Verification items for the finished model (mm, model axes). A direction names the side the tool comes from. Give positions to 0.01 mm unless a question says otherwise; leave off trailing zeros. Order: outer loops, then holes, each group sorted by start corner. A loop starts at its lowest first (then second) coordinate and runs counter-clockwise, first axis right, second up.
(1) Sectioned sample at D-D on z = -23. Record the cut outline in (x, y).
(2) Sectioned sample at B-B on y = 0. Record the cut outline in (x, z), plus the area to 3 significant figures.
(3) Sectioned sample at C-C on z = -9. Record the cut outline in (x, y).
(4) Scan lines: L1, parallel to Y at x = -11.6, z = -8; L2, parallel to Y at x = -10.05, z = -8.5; L3, parallel to Y at x = -11.4, z = 1. Record each from-to range of solid material in increasing order.
(5) Mould release check, pull along Z, two halves, no side actions. Record for faces 1 (the face through (-11, -11, -6.201)), 2 (the face through (-11, 0, -37)), 3 (the face through (-11, 9.615, 25)), 4 (the face through (-10, 0, 38)): pulls with the +Z half, pulls with the -Z half, needs draft (parallel to the pull), parting line crosses it, or undercut.
(6) Gauge pin test, flat ends, axial feed: pin 1 (5 mm diameter, centred on y = 12.5, z = 11.5, fed in from -X); pin 2 (0.9 mm diameter, centred on x = -10, z = 1.5, fed in from +Y); pin 3 (1.5 mm diameter, centred on x = -11, y = -11.5, fed in from -Z); pin 4 (0.9 mm diameter, centred on x = -10.5, y = 15.5, fed in from +Z). Record the tip position at first contact, or that the pin passes through.
(7) Sectioned sample at A-A on z = -0.5. Record the cut outline in (x, y), plus the area to 3 significant figures.
(8) Access from +Z, -Z, +X, -X, +Y, -Y to the whole of each face (thin tool, end or side, straight path). Record for faces 5 (the face through (-11, -13.215, -12)), 6 (the face through (-9.986, 3.007, 21.603)), 7 (the face through (-11, -2, 0)), 8 (the face through (-10.521, 12.915, -5.256)), 9 (the face through (-11, 10, 16.024)).
```python
from build123d import *
from build123d.topology import SkipClean

# Parameters (mm, degrees)
BOSS_EXTRUDE1_DEPTH      = 7
BOSS_EXTRUDE1_DEPTH_BACK = 7
SKETCH3_R                = 7
BOSS_EXTRUDE2_DEPTH      = 3
CUT_EXTRUDE1_DEPTH       = 23
CUT_EXTRUDE1_DEPTH_BACK  = 23
SKETCH4_R                = 4
BOSS_EXTRUDE3_DEPTH      = 3
CUT_EXTRUDE2_DEPTH       = 20
CUT_EXTRUDE2_DEPTH_BACK  = 30
SKETCH6_W                = 36.146068324
SKETCH6_H                = 79.881394618
SKETCH7_W                = 6
SKETCH7_H                = 2
BOSS_EXTRUDE4_DEPTH      = 25
SKETCH8_R                = 1.5
CUT_EXTRUDE3_DEPTH       = 25
SKETCH9_W                = 6
SKETCH9_H                = 2
BOSS_EXTRUDE5_DEPTH      = 11
SKETCH10_R               = 4
SKETCH10_R_2             = 3.65
BOSS_EXTRUDE7_DEPTH      = 3
SKETCH11_R               = 2.4
CUT_EXTRUDE4_DEPTH       = 3
BOSS_EXTRUDE9_START      = -1
SKETCH13_W               = 69.204545587
SKETCH13_H               = 9.322892152
SKETCH13_R               = 3.65
BOSS_EXTRUDE9_DEPTH      = 1
SKETCH14_W               = 11.115756027
SKETCH14_H               = 43.925164946
CUT_EXTRUDE5_DEPTH       = 31
CUT_EXTRUDE6_DEPTH       = 22
SKETCH16_W               = 30.440127373
SKETCH16_H               = 8.446463946
CUT_EXTRUDE7_DEPTH       = 10
SKETCH17_W               = 7
SKETCH17_H               = 4
CUT_EXTRUDE8_DEPTH       = 10


with BuildPart() as part:
    # Sketch2 → Boss-Extrude1 (new, two sides: drawn at the far end of the back side and taken through both)
    with BuildSketch(Plane(origin=(0, 0, 0), x_dir=(1, 0, 0), z_dir=(0, 1, 0)).offset(-BOSS_EXTRUDE1_DEPTH_BACK)):
        Polygon((12, 30), (12, -30), (9, -30), (9, -1.5), (-9, -1.5), (-9, -30), (-12, -30), (-12, 30), (-9, 30), (-9, 1.5), (9, 1.5), (9, 30), align=None)
    extrude(amount=BOSS_EXTRUDE1_DEPTH + BOSS_EXTRUDE1_DEPTH_BACK)

    # Sketch3 → Boss-Extrude2 (add)
    with BuildSketch(Plane(origin=(12, 0, 0), x_dir=(0, 0, -1), z_dir=(1, 0, 0))):
        with Locations((-30, 0)):
            Circle(SKETCH3_R)
        with Locations((30, 0)):
            Circle(SKETCH3_R)
    boss_extrude2 = extrude(amount=-BOSS_EXTRUDE2_DEPTH)

    # Mirror1: Boss-Extrude2 across plane
    add(boss_extrude2.mirror(Plane.ZY))

    # Sketch4 → Cut-Extrude1 (cut, two sides: drawn at the far end of the back side and taken through both)
    with BuildSketch(Plane.ZY.offset(-CUT_EXTRUDE1_DEPTH_BACK)):
        with Locations(Location((-30, 0, 0), (0, 0, 180))):
            Circle(SKETCH4_R)
        with Locations(Location((30, 0, 0), (0, 0, 180))):
            Circle(SKETCH4_R)
    extrude(amount=CUT_EXTRUDE1_DEPTH + CUT_EXTRUDE1_DEPTH_BACK, mode=Mode.SUBTRACT)

    # Sketch5 → Boss-Extrude3 (add)
    with BuildSketch(Plane.ZY.offset(12)):
        Polygon((-30, 7), (-24.155374342, 13.339180653), (-3.984430585, 16.782248387), (-3.984430585, 13.558363221), (-6.564031008, 12.252853794), (-9.961076462, 7), align=None)
        Polygon((5.630173652, 7), (6.872920148, 8.921659787), (16.024340395, 8.921659787), (16.024340395, 11.520201473), (23.010764714, 11.520201473), (24.017423371, 9.614604237), (26.442728945, 9.614604237), (25.802127981, 10.827257024), (33.625376893, 10.827257024), (39.584451678, 2.208760433), (39.584451678, -0.649635421), (35.450408088, -0.649635421), (35.450408088, 3.248177107), (30.561687085, 6.409736158), (5.630173652, 6.409736158), align=None)
        Polygon((-30, -7), (-17.229678236, -13.21512033), (-6.200995871, -13.21512033), (-6.200995871, -8.829973728), (-9.961076462, -7), align=None)
        Polygon((9.961076462, -7), (15.524820582, -9.707789187), (15.524820582, -13.295871625), (32.135298846, -13.295871625), (32.135298846, -11.501830406), (39.584451678, -7), (39.584451678, -3.334795163), (35.450408088, -3.334795163), (31.744983073, -5.574136385), (9.961076462, -5.574136385), align=None)
    boss_extrude3 = extrude(amount=-BOSS_EXTRUDE3_DEPTH)

    # Mirror2: Boss-Extrude3 across plane
    add(boss_extrude3.mirror(Plane.ZY))

    # Sketch6 → Cut-Extrude2 (cut, two sides: drawn at the far end of the back side and taken through both)
    with BuildSketch(Plane(origin=(0, 7, 0), x_dir=(1, 0, 0), z_dir=(0, 1, 0)).offset(-CUT_EXTRUDE2_DEPTH_BACK)):
        with Locations((9.073034162, -2.940697309)):
            Rectangle(SKETCH6_W, SKETCH6_H)
    extrude(amount=CUT_EXTRUDE2_DEPTH + CUT_EXTRUDE2_DEPTH_BACK, mode=Mode.SUBTRACT)

    # Sketch7 → Boss-Extrude4 (add)
    with BuildSketch(Plane.ZY.offset(12)):
        with Locations((0, -2)):
            Rectangle(SKETCH7_W, SKETCH7_H)
    extrude(amount=BOSS_EXTRUDE4_DEPTH)

    # Sketch8 → Cut-Extrude3 (cut)
    with BuildSketch(Plane(origin=(0, -1, 0), x_dir=(1, 0, 0), z_dir=(0, 1, 0))):
        with Locations(Location((-34, 0, 0), (0, 0, 270))):
            Circle(SKETCH8_R)
        with Locations(Location((-26, 0, 0), (0, 0, 270))):
            Circle(SKETCH8_R)
    extrude(amount=-CUT_EXTRUDE3_DEPTH, mode=Mode.SUBTRACT)

    # Sketch9 → Boss-Extrude5 (add)
    with BuildSketch(Plane.ZY.offset(12)):
        Rectangle(SKETCH9_W, SKETCH9_H)
    extrude(amount=BOSS_EXTRUDE5_DEPTH)

    # Sketch10 → Boss-Extrude7 (add)
    # profile 1 of 2: a face of its own
    with BuildSketch(Plane(origin=(-9, 0, 0), x_dir=(0, 0, -1), z_dir=(1, 0, 0))):
        with Locations((-30, 0)):
            Circle(SKETCH10_R)
        with Locations((-30, 0)):
            Circle(SKETCH10_R_2, mode=Mode.SUBTRACT)
    # profile 2 of 2: a face of its own
    with BuildSketch(Plane(origin=(-9, 0, 0), x_dir=(0, 0, -1), z_dir=(1, 0, 0))):
        with Locations((30, 0)):
            Circle(SKETCH10_R)
        with Locations((30, 0)):
            Circle(SKETCH10_R_2, mode=Mode.SUBTRACT)
    extrude(amount=-BOSS_EXTRUDE7_DEPTH)

    # Sketch11 → Cut-Extrude4 (cut)
    with BuildSketch(Plane(origin=(-9, 0, 0), x_dir=(0, 0, -1), z_dir=(1, 0, 0))):
        with BuildLine():
            Line((-13.713664596, 2.392755549), (-29.716614907, 3.638982397))
            ThreePointArc((-29.716614907, 3.638982397), (-27.320741186, 2.478723907), (-26.35, 0))
            ThreePointArc((-26.35, 0), (-27.320741186, -2.478723907), (-29.716614907, -3.638982397))
            Line((-29.716614907, -3.638982397), (-13.713664596, -2.392755549))
            ThreePointArc((-13.713664596, -2.392755549), (-16.3, 0), (-13.713664596, 2.392755549))
        make_face()
        with Locations((-13.9, 0)):
            Circle(SKETCH11_R)
        with BuildLine():
            Line((29.716614907, 3.638982397), (13.713664596, 2.392755549))
            ThreePointArc((13.713664596, 2.392755549), (15.529845856, 1.761704426), (16.3, 0))
            ThreePointArc((16.3, 0), (15.529845856, -1.761704426), (13.713664596, -2.392755549))
            Line((13.713664596, -2.392755549), (29.716614907, -3.638982397))
            ThreePointArc((29.716614907, -3.638982397), (26.35, 0), (29.716614907, 3.638982397))
        make_face()
        with Locations((13.9, 0)):
            Circle(SKETCH11_R)
    extrude(amount=-CUT_EXTRUDE4_DEPTH, mode=Mode.SUBTRACT)

    # Sketch13 → Boss-Extrude9 (add)
    with SkipClean():  # the faces are left unmerged after this step: merging them gives an invalid solid
        with BuildSketch(Plane.ZY.offset(12).offset(BOSS_EXTRUDE9_START)):
            with Locations((0.485437096, -0.184140285)):
                Rectangle(SKETCH13_W, SKETCH13_H)
            with Locations(Location((-30, 0, 0), (0, 0, 85.547088609))):
                Circle(SKETCH13_R, mode=Mode.SUBTRACT)
            with Locations(Location((30, 0, 0), (0, 0, 265.547088609))):
                Circle(SKETCH13_R, mode=Mode.SUBTRACT)
        extrude(amount=BOSS_EXTRUDE9_DEPTH)
    add(part.part.scale(1), mode=Mode.REPLACE)  # the faces are merged on a copy

    # Sketch14 → Cut-Extrude5 (cut)
    with BuildSketch(Plane(origin=(-9, 0, 0), x_dir=(0, 0, -1), z_dir=(1, 0, 0))):
        with Locations((-43.557878014, -0.721999448)):
            Rectangle(SKETCH14_W, SKETCH14_H)
    extrude(amount=-CUT_EXTRUDE5_DEPTH, mode=Mode.SUBTRACT)

    # Sketch15 → Cut-Extrude6 (cut)
    with BuildSketch(Plane(origin=(-9, 0, 0), x_dir=(0, 0, -1), z_dir=(1, 0, 0))):
        Polygon((-39.300223418, -0.896828093), (-32.576713138, 8.827257024), (-29.273128497, 8.827257024), (-29.273128497, 11.015866037), (-39.300223418, 11.015866037), align=None)
    extrude(amount=-CUT_EXTRUDE6_DEPTH, mode=Mode.SUBTRACT)

    # Sketch16 → Cut-Extrude7 (cut)
    with BuildSketch(Plane(origin=(0, 1, 0), x_dir=(1, 0, 0), z_dir=(0, 1, 0))):
        with Locations((-27.220063687, 1.223231973)):
            Rectangle(SKETCH16_W, SKETCH16_H)
    extrude(amount=-CUT_EXTRUDE7_DEPTH, mode=Mode.SUBTRACT)

    # Sketch17 → Cut-Extrude8 (cut)
    with BuildSketch(Plane.ZY.offset(12)):
        Rectangle(SKETCH17_W, SKETCH17_H)
    extrude(amount=-CUT_EXTRUDE8_DEPTH, mode=Mode.SUBTRACT)


solid = part.part
```
Ans:
1. outline: (-12, -10.41) - (-9, -10.41) - (-9, -3.12) - (-11, -3.12) - (-11, 3.12) - (-9, 3.12) - (-9, 13.54) - (-12, 13.54) - close
2. outline: (-12, -37) - (-9, -37) - (-9, -33.65) - (-12, -33.65) - close; (-12, -26.35) - (-11, -26.35) - (-11, -11.5) - (-9, -11.5) - (-9, -3.5) - (-12, -3.5) - close; (-12, 3.5) - (-9, 3.5) - (-9, 11.5) - (-11, 11.5) - (-11, 26.35) - (-12, 26.35) - close; (-12, 33.65) - (-9, 33.65) - (-9, 38) - (-12, 38) - close
2. area: 101 mm2
3. outline: (-12, -13.22) - (-9, -13.22) - (-9, -7.47) - (-12, -7.47) - close; (-12, -7) - (-9, -7) - (-9, 7) - (-12, 7) - close; (-12, 8.49) - (-9, 8.49) - (-9, 15.93) - (-12, 15.93) - close
4. L1: y = -13.22 to -7.95, -7 to 7, 10.03 to 16.1
4. L2: y = -13.22 to -7.71, -7 to 7, 9.26 to 16.01
4. L3: y = -7 to -2, 2 to 7
5. face 1: undercut
5. face 2: pulls with the -Z half
5. face 3: undercut
5. face 4: pulls with the +Z half
6. pin 1: passes through
6. pin 2: stops at y = 7
6. pin 3: stops at z = -22.29
6. pin 4: stops at z = -3.98
7. outline: (-12, -7) - (-9, -7) - (-9, -2) - (-12, -2) - close; (-12, 2) - (-9, 2) - (-9, 7) - (-12, 7) - close
7. area: 30.0 mm2
8. face 5: -Z, +X, -X, -Y
8. face 6: +X
8. face 7: +X, -X
8. face 8: +Z, +X, -X
8. face 9: +X, -X, +Y
